Model file for the job. Use its own axes, mm. Give positions to 0.01 mm unless a question says otherwise; leave off trailing zeros. Loops run counter-clockwise (first coordinate to the right, second up) from the corner with the lowest first, then second, coordinate; pieces in that order, holes last. Notation, with made-up numbers: (27.5, 43) - (83.5, 43) arc R21 ccw to (83.5, 82) - close; hole circle Ø4 at (5.5, 79). An arc over 180 degrees is marked (long way). Use a Markdown table: item, result.
from build123d import *

# Parameters (mm, degrees)
SKETCH_1_R          = 1.462780711
SKETCH_1_R_2        = 1.582906388
SKETCH_1_R_3        = 1.5
SKETCH_1_R_4        = 1.65
EXTRUDE_1_DEPTH     = 4
SKETCH_3_R          = 3.5
SKETCH_3_R_2        = 1.6
CUT_EXTRUDE_1_DEPTH = 4
SKETCH_4_R          = 4.5
SKETCH_4_R_2        = 2.1
CUT_EXTRUDE_2_DEPTH = 4
CUT_EXTRUDE_7_DEPTH = 4
SKETCH_12_W         = 118
SKETCH_12_H         = 10
CUT_EXTRUDE_8_DEPTH = 4
SKETCH_13_W         = 20
SKETCH_13_H         = 15
SKETCH_13_R         = 1.6
EXTRUDE_4_DEPTH     = 4
FILLET_4_R          = 3


with BuildPart() as part:
    # 草图1 → 凸台-拉伸1 (new body)
    with BuildSketch(Plane.XY):
        Polygon((-128, 10), (-128, -10), (-10, -128), (10, -128), (10, 10), align=None)
        with Locations((-44.314491387, -77.548510103)):
            Circle(SKETCH_1_R, mode=Mode.SUBTRACT)
        with Locations((-38.657637138, -71.891655854)):
            Circle(SKETCH_1_R_2, mode=Mode.SUBTRACT)
        with Locations((-77.548510103, -44.314491387)):
            Circle(SKETCH_1_R_3, mode=Mode.SUBTRACT)
        with Locations((-71.891655854, -38.657637138)):
            Circle(SKETCH_1_R_3, mode=Mode.SUBTRACT)
        with Locations((-29.196699141, -46.874368671)):
            Circle(SKETCH_1_R_4, mode=Mode.SUBTRACT)
        with Locations((-46.874368671, -29.196699141)):
            Circle(SKETCH_1_R_4, mode=Mode.SUBTRACT)
        with Locations((-22.125631329, -39.803300859)):
            Circle(SKETCH_1_R_4, mode=Mode.SUBTRACT)
        with Locations((-39.803300859, -22.125631329)):
            Circle(SKETCH_1_R_4, mode=Mode.SUBTRACT)
    extrude(amount=EXTRUDE_1_DEPTH)

    # 草图3 → 切除-拉伸1 (cut)
    with BuildSketch(Plane.XY.offset(4)):
        Circle(SKETCH_3_R)
        with Locations((5, 5)):
            Circle(SKETCH_3_R_2)
        with Locations((-5, 5)):
            Circle(SKETCH_3_R_2)
        with Locations((-5, -5)):
            Circle(SKETCH_3_R_2)
        with Locations((5, -5)):
            Circle(SKETCH_3_R_2)
        with Locations((-20, -5)):
            Circle(SKETCH_3_R_2)
        with Locations((-5, -20)):
            Circle(SKETCH_3_R_2)
        with Locations((5, -20)):
            Circle(SKETCH_3_R_2)
        with Locations((5, 20)):
            Circle(SKETCH_3_R_2)
        with Locations((-5, 20)):
            Circle(SKETCH_3_R_2)
        with Locations((20, -5)):
            Circle(SKETCH_3_R_2)
        with Locations((20, 5)):
            Circle(SKETCH_3_R_2)
        with Locations((-20, 5)):
            Circle(SKETCH_3_R_2)
    extrude(amount=-CUT_EXTRUDE_1_DEPTH, mode=Mode.SUBTRACT)

    # 草图4 → 切除-拉伸2 (cut)
    with BuildSketch(Plane.XY.offset(4)):
        with Locations((0, -60)):
            Circle(SKETCH_4_R)
        with Locations((-5, -29.263884189)):
            Circle(SKETCH_4_R_2)
        with Locations((5, -29.263884189)):
            Circle(SKETCH_4_R_2)
        with Locations((5, -49.263884189)):
            Circle(SKETCH_4_R_2)
        with Locations((5, -69.263884189)):
            Circle(SKETCH_4_R_2)
        with Locations((5, -89.263884189)):
            Circle(SKETCH_4_R_2)
        with Locations((-5, -49.263884189)):
            Circle(SKETCH_4_R_2)
        with Locations((-5, -69.263884189)):
            Circle(SKETCH_4_R_2)
        with Locations((-5, -89.263884189)):
            Circle(SKETCH_4_R_2)
        with Locations(Location((-89.263884189, -5, 0), (0, 0, 180))):
            Circle(SKETCH_4_R_2)
        with Locations(Location((-69.263884189, -5, 0), (0, 0, 180))):
            Circle(SKETCH_4_R_2)
        with Locations(Location((-49.263884189, -5, 0), (0, 0, 180))):
            Circle(SKETCH_4_R_2)
        with Locations(Location((-89.263884189, 5, 0), (0, 0, 180))):
            Circle(SKETCH_4_R_2)
        with Locations(Location((-69.263884189, 5, 0), (0, 0, 180))):
            Circle(SKETCH_4_R_2)
        with Locations(Location((-49.263884189, 5, 0), (0, 0, 180))):
            Circle(SKETCH_4_R_2)
        with Locations(Location((-29.263884189, 5, 0), (0, 0, 180))):
            Circle(SKETCH_4_R_2)
        with Locations(Location((-29.263884189, -5, 0), (0, 0, 180))):
            Circle(SKETCH_4_R_2)
        with Locations(Location((-60, 0, 0), (0, 0, 180))):
            Circle(SKETCH_4_R)
    extrude(amount=-CUT_EXTRUDE_2_DEPTH, mode=Mode.SUBTRACT)

    # 草图11 → 切除-拉伸7 (cut)
    with BuildSketch(Plane.XY.offset(4)):
        Polygon((-69, -69), (-64.050252532, -64.050252532), (-99.405591591, -28.694913472), (-104.355339059, -33.644660941), align=None)
        Polygon((-28.694913472, -99.405591591), (-64.050252532, -64.050252532), (-69, -69), (-33.644660941, -104.355339059), align=None)
    extrude(amount=-CUT_EXTRUDE_7_DEPTH, mode=Mode.SUBTRACT)

    # 草图12 → 切除-拉伸8 (cut)
    with BuildSketch(Plane.XY.offset(4)):
        with Locations((-69, 5)):
            Rectangle(SKETCH_12_W, SKETCH_12_H)
    extrude(amount=-CUT_EXTRUDE_8_DEPTH, mode=Mode.SUBTRACT)

    # 草图13 → 凸台-拉伸4 (add)
    with BuildSketch(Plane.XY.offset(4)):
        with Locations((0, 17.5)):
            Rectangle(SKETCH_13_W, SKETCH_13_H)
        with Locations((-5, 20)):
            Circle(SKETCH_13_R, mode=Mode.SUBTRACT)
        with Locations((5, 20)):
            Circle(SKETCH_13_R, mode=Mode.SUBTRACT)
    extrude(amount=-EXTRUDE_4_DEPTH)

    # 圆角4
    fillet_4_edges = [part.edges().sort_by_distance(p)[0] for p in [
        (-99.405591591, -28.694913472, 2),
        (-28.694913472, -99.405591591, 2),
        (-33.644660941, -104.355339059, 2),
        (-104.355339059, -33.644660941, 2),
        (-64.5, 0, 2),
        (-55.5, 0, 2),
        (-10, 0, 2),
        (-128, 0, 2),
        (10, -128, 2),
        (-10, -128, 2),
        (-128, -10, 2),
        (10, 25, 2),
        (-10, 25, 2),
    ]]
    fillet(fillet_4_edges, radius=FILLET_4_R)


solid = part.part
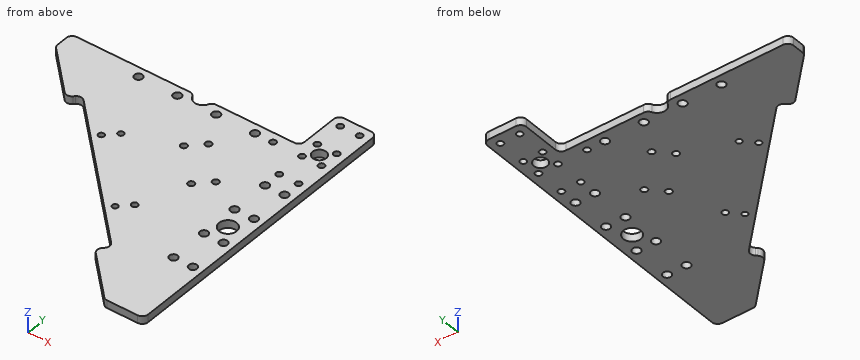
(1) Slice it at B-B, the plane z = 0.8. Count the separate pieces of the cut face and the enclosed holes in it, plus the area to 3 significant figures.
Computed:
| item | result |
|---|---|
| separate pieces | 1 |
| enclosed holes | 31 |
| area | 10,100 mm² |
(2) Slice it at A-A, the plane x = -89.5. Write the cut outline in (y, z).
Computed:
| item | result |
|---|---|
| outline | (-38.6, 0) - (-7.09, 0) - (-7.09, 4) - (-38.6, 4) - close; (-2.91, 0) - (0, 0) - (0, 4) - (-2.91, 4) - close |
(3) Drill centre lines: probe 1 along X at (y, z) = (7.5, 3.6); probe 2 along X at (y, z) = (-67.5, 1.9); probe 3 along X at (y, z) = (-46.5, 1.9). Where is each one in solid material? Low to high. Write a range as [from, to].
Computed:
| item | result |
|---|---|
| probe 1 | [-10, 10] |
| probe 2 | [-60.6, -6.14], [-3.86, 3.86], [6.14, 10] |
| probe 3 | [-81.6, -30.8], [-27.59, 10] |
